Geometry: see drawing. Coordinates: mm, zero at the bounding-box minimum. Give positions to 0.01 mm unless a question says otherwise; leave off trailing zeros. Order: outer loops, then holes, each group sorted by start corner. A loop starts at its lowest first (then second) coordinate and runs counter-clockwise, first axis right, second up. Notation, with made-up numbers: M 65,47 L 91,47 A38 cw 91,85 Z; hole C -30,1.25 d3. An arc over 180 degrees is marked long. Return JSON: item names as keys, results as strings.
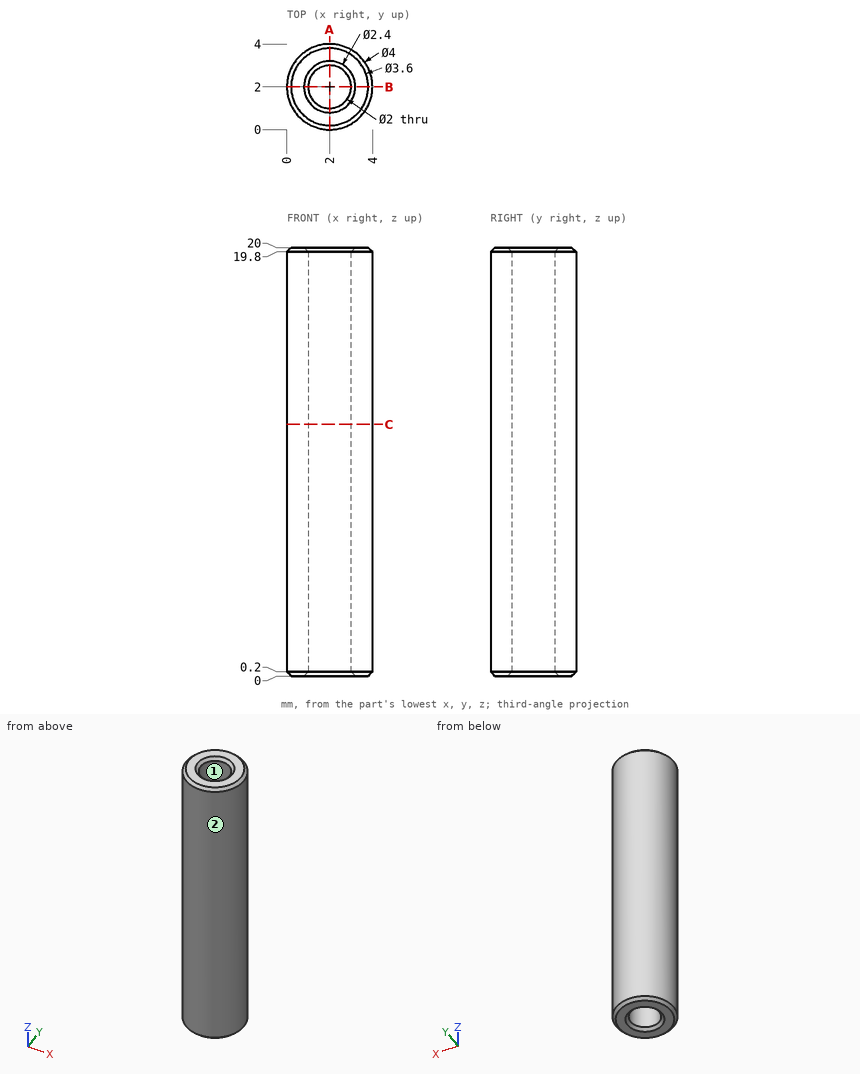
1. First-contact query: pin 1 (1.5 mm diameter, centred on x = 1, z = 16, fed in from +Y). Flat tip, straight axial feed; report the tip coordinate or a pass-through.
Evaluation:
{"pin 1": "stops at y = 3.98"}
2. Section query A-A (x = 2). Return loops of the section in (y, z).
Evaluation:
{"outline": "M 0,0.2 L 0.2,0 L 0.8,0 L 1,0.2 L 1,19.8 L 0.8,20 L 0.2,20 L 0,19.8 Z; M 3,0.2 L 3.2,0 L 3.8,0 L 4,0.2 L 4,19.8 L 3.8,20 L 3.2,20 L 3,19.8 Z"}
3. Ray query, probe 1 along X at (y, z) = (2.1, 1); probe 2 along Y at (x, z) = (2, 15); probe 3 along Y at (x, z) = (2.45, 15.5). Return the intervals inside material, ascending.
Evaluation:
{"probe 1": "x = 0 to 1.01, 2.99 to 4", "probe 2": "y = 0 to 1, 3 to 4", "probe 3": "y = 0.05 to 1.11, 2.89 to 3.95"}
4. Section query C-C (z = 11.75). Return loops of the section in (x, y).
Evaluation:
{"outline": "C 2,2 d4; hole C 2,2 d2"}
5. Draft query along Y for the marked faces 1 and 2. Return one class per face: pulls with the +Y half, pulls with the -Y half, needs draft (parallel to the pull), parting line crosses it, or undercut.
Evaluation:
{"face 1": "undercut", "face 2": "parting line crosses it"}
